Verification items for the finished model (mm, model axes). A direction names the side the tool comes from. Coordinates: 2 decimals unless noted, no trailing zeros. Order: outer loops, then holes, each group sorted by start corner. A loop starts at its lowest first (then second) coordinate and runs counter-clockwise, first axis right, second up. Notation, with made-up numbers: M -39.5,45 L 0.5,45 A15 ccw 0.5,65 Z; hole C 72.25,37 d5. An arc over 180 degrees is marked long. Use one line per item in the form item = value. Start each with the question number.
```python
from build123d import *

# Parameters (mm, degrees)
SKETCH1_W                 = 50
SKETCH1_H                 = 30
BOSS_EXTRUDE1_DEPTH       = 7
SKETCH2_W                 = 27
SKETCH2_H                 = 60.3
BOSS_EXTRUDE2_DEPTH       = 5
SKETCH3_W                 = 40
SKETCH3_H                 = 7
BOSS_EXTRUDE3_DEPTH       = 12
SKETCH4_R                 = 6.65
CUT_EXTRUDE1_DEPTH        = 4
CUT_EXTRUDE2_REACH        = 96.439
SKETCH5_R                 = 2.9
SKETCH6_W                 = 8
SKETCH6_H                 = 10
CUT_EXTRUDE3_DEPTH        = 93.681659459
F_2_CLEARANCE_HOLE1_D     = 2.7051
F_2_CLEARANCE_HOLE1_DEPTH = 8
SKETCH10_W                = 50
SKETCH10_H                = 7
BOSS_EXTRUDE4_DEPTH       = 2
SKETCH11_W                = 5
SKETCH11_H                = 53.3
BOSS_EXTRUDE5_DEPTH       = 2
SKETCH13_W                = 5
SKETCH13_H                = 6.35
BOSS_EXTRUDE6_DEPTH       = 30
SKETCH14_W                = 30
SKETCH14_H                = 6.35
BOSS_EXTRUDE7_DEPTH       = 40
SKETCH15_W                = 28.462792601
SKETCH15_H                = 7
CUT_EXTRUDE4_DEPTH        = 93.681659459
SKETCH16_W                = 3.81
SKETCH16_H                = 34.732
CUT_EXTRUDE5_DEPTH        = 93.681659459


with BuildPart() as part:
    # Sketch1 → Boss-Extrude1 (new body)
    with BuildSketch(Plane(origin=(0, 0, 0), x_dir=(1, 0, 0), z_dir=(0, 1, 0))):
        with Locations((25, 15)):
            Rectangle(SKETCH1_W, SKETCH1_H)
    extrude(amount=BOSS_EXTRUDE1_DEPTH)

    # Sketch2 → Boss-Extrude2 (add)
    with BuildSketch(Plane(origin=(50, 0, 0), x_dir=(0, 0, -1), z_dir=(1, 0, 0))):
        with Locations((43.5, -23.15)):
            Rectangle(SKETCH2_W, SKETCH2_H)
    boss_extrude2 = extrude(amount=-BOSS_EXTRUDE2_DEPTH)

    # Mirror1: Boss-Extrude2 across plane
    add(boss_extrude2.mirror(Plane(origin=(25, 0, 0), x_dir=(0, 0, 1), z_dir=(1, 0, 0))))

    # Sketch3 → Boss-Extrude3 (add)
    with BuildSketch(Plane(origin=(0, 0, -30), x_dir=(-1, 0, 0), z_dir=(0, 0, -1))):
        with Locations((-25, 3.5)):
            Rectangle(SKETCH3_W, SKETCH3_H)
    extrude(amount=BOSS_EXTRUDE3_DEPTH)

    # Sketch4 → Cut-Extrude1 (cut)
    with BuildSketch(Plane(origin=(0, 7, 0), x_dir=(1, 0, 0), z_dir=(0, 1, 0))):
        with Locations(Location((25, 34, 0), (0, 0, 270))):
            Circle(SKETCH4_R)
    extrude(amount=-CUT_EXTRUDE1_DEPTH, mode=Mode.SUBTRACT)

    # Sketch5 → Cut-Extrude2 (cut, up to next)
    with BuildSketch(Plane(origin=(0, 3, 0), x_dir=(1, 0, 0), z_dir=(0, 1, 0)), mode=Mode.PRIVATE) as cut_extrude2_sk1:
        with Locations(Location((25, 34, 0), (0, 0, 270))):
            Circle(SKETCH5_R)
    cut_extrude2_tool1 = extrude(cut_extrude2_sk1.sketch, amount=-CUT_EXTRUDE2_REACH, mode=Mode.PRIVATE) & part.part
    add(cut_extrude2_tool1.solids().sort_by_distance((25, 3, -34))[0], mode=Mode.SUBTRACT)

    # Sketch6 → Cut-Extrude3 (cut, through all)
    with BuildSketch(Plane(origin=(50, 0, 0), x_dir=(0, 0, -1), z_dir=(1, 0, 0))):
        with Locations((45, -8)):
            Rectangle(SKETCH6_W, SKETCH6_H)
        with Locations((45, -38.3)):
            Rectangle(SKETCH6_W, SKETCH6_H)
    extrude(amount=-CUT_EXTRUDE3_DEPTH, mode=Mode.SUBTRACT)

    # #2 Clearance Hole1
    with Locations(Plane.XY.offset(-49)):
        with Locations((47.5, -38.3), (47.5, -8), (2.5, -8), (2.5, -38.3)):
            Hole(F_2_CLEARANCE_HOLE1_D / 2, depth=F_2_CLEARANCE_HOLE1_DEPTH)

    # Sketch10 → Boss-Extrude4 (add)
    with BuildSketch(Plane.XY):
        with Locations((25, 3.5)):
            Rectangle(SKETCH10_W, SKETCH10_H)
    extrude(amount=BOSS_EXTRUDE4_DEPTH)

    # Sketch11 → Boss-Extrude5 (add)
    with BuildSketch(Plane.XY.offset(-30)):
        with Locations((47.5, -26.65)):
            Rectangle(SKETCH11_W, SKETCH11_H)
        with Locations((2.5, -26.65)):
            Rectangle(SKETCH11_W, SKETCH11_H)
    extrude(amount=BOSS_EXTRUDE5_DEPTH)

    # Sketch13 → Boss-Extrude6 (add)
    with BuildSketch(Plane.XY.offset(-28)):
        with Locations((47.5, -15.393)):
            Rectangle(SKETCH13_W, SKETCH13_H)
        with Locations((2.5, -15.393)):
            Rectangle(SKETCH13_W, SKETCH13_H)
    extrude(amount=BOSS_EXTRUDE6_DEPTH)

    # Sketch14 → Boss-Extrude7 (add)
    with BuildSketch(Plane.ZY.offset(-45)):
        with Locations((-13, -15.393)):
            Rectangle(SKETCH14_W, SKETCH14_H)
    extrude(amount=BOSS_EXTRUDE7_DEPTH)

    # Sketch15 → Cut-Extrude4 (cut, through all)
    with BuildSketch(Plane(origin=(50, 0, 0), x_dir=(0, 0, -1), z_dir=(1, 0, 0))):
        with Locations((12.231396301, 3.5)):
            Rectangle(SKETCH15_W, SKETCH15_H)
    extrude(amount=-CUT_EXTRUDE4_DEPTH, mode=Mode.SUBTRACT)

    # Sketch16 → Cut-Extrude5 (cut, through all)
    with BuildSketch(Plane(origin=(50, 0, 0), x_dir=(0, 0, -1), z_dir=(1, 0, 0))):
        with Locations((29.905, -35.934)):
            Rectangle(SKETCH16_W, SKETCH16_H)
    extrude(amount=-CUT_EXTRUDE5_DEPTH, mode=Mode.SUBTRACT)


solid = part.part
```
1. Cross-section at D-D on y = -38.3. Enter the section's corners in (x, z), and give its area (3 significant figures).
2. Depth check by flat-ended pin: P1, Ø12, axis at x = 10.5, y = -22.5, coming from the -Z side; P2, Ø6.5, axis at x = 25, z = -34, coming from the -Y side; P3, Ø2.5, axis at x = 2, y = -43.5, coming from the +Z side; P4, Ø3, axis at x = 47.5, y = -8, coming from the +Z side. Enter the tip coordinate at first touch or a pass-through.
3. Release check for a two-part mould opening along Y. For faces 4 (the flat face through (25, 4, -42)), 5 (the cylindrical face through (1.77, -6.86, -53.06)), 6 (the flat face through (47, -53.3, -45)), 7 (the flat face through (48, -8, -41)) record: pulls with the +Y half, pulls with the -Y half, needs draft (parallel to the pull), parting line crosses it, or undercut.
4. Tool access check on faces 1 (the cylindrical face through (2.68, -36.96, -53.06)), 2 (the flat face through (49, -9, -49)), 3 (the flat face through (22, 3, -33)). Record the directions out of +Z, -Z, +X, -X, +Y, -Y that give a thin tool (end or side, any length) a straight path to the whole face; none if there is none.
5. Cross-section at B-B on x = 39. Enter the section's corners in (y, z), and give its area (3 significant figures).
6. Cross-section at C-C on z = -47. Enter the section's corners in (x, y), and give its area (3 significant figures).
7. Cross-section at A-A on y = -48.5. Enter the section's corners in (x, z).
8. Material ranges on line 1 along X through (y, z) = (-38, -50); line 2 along Y through (x, z) = (2, -51); line 3 along X through (y, z) = (-19.5, -53.5), recorded low to high.
Final values:
q1.outline = M 0,-57 L 1.15,-57 L 1.15,-49 L 0,-49 Z; M 0,-41 L 5,-41 L 5,-31.81 L 0,-31.81 Z; M 3.85,-57 L 5,-57 L 5,-49 L 3.85,-49 Z; M 45,-57 L 46.15,-57 L 46.15,-49 L 45,-49 Z; M 45,-41 L 50,-41 L 50,-31.81 L 45,-31.81 Z; M 48.85,-57 L 50,-57 L 50,-49 L 48.85,-49 Z
q1.area = 129 mm2
q2.P1 = -57
q2.P2 = 0
q2.P3 = -31.81
q2.P4 = -28
q3.face_4 = needs draft
q3.face_5 = undercut
q3.face_6 = pulls with the -Y half
q3.face_7 = undercut
q4.face_1 = -Z
q4.face_2 = +X, -X
q4.face_3 = +Y
q5.outline = M -18.57,-28 L -12.22,-28 L -12.22,2 L -18.57,2 Z; M 0,-42 L 7,-42 L 7,-26.46 L 0,-26.46 Z
q5.area = 299 mm2
q6.outline = M 0,-53.3 L 5,-53.3 L 5,-43.3 L 0,-43.3 Z; M 0,-33.3 L 5,-33.3 L 5,-13 L 0,-13 Z; M 0,-3 L 5,-3 L 5,7 L 0,7 Z; M 45,-53.3 L 50,-53.3 L 50,-43.3 L 45,-43.3 Z; M 45,-33.3 L 50,-33.3 L 50,-13 L 45,-13 Z; M 45,-3 L 50,-3 L 50,7 L 45,7 Z
q6.area = 403 mm2
q7.outline = M 0,-57 L 5,-57 L 5,-31.81 L 0,-31.81 Z; M 45,-57 L 50,-57 L 50,-31.81 L 45,-31.81 Z
q8.line_1 = 0 to 1.18, 3.82 to 5, 45 to 46.18, 48.82 to 50
q8.line_2 = -53.3 to -39.56, -37.04 to -9.26, -6.74 to 7
q8.line_3 = 0 to 5, 45 to 50
